Work out the finished part from the listing and answer in its coordinate system (mm). Face numbers are marked on the shaded views. A direction names the side the tool comes from. Round coordinates to 2 decimals unless told otherwise and drop trailing zeros. Loops run counter-clockwise (first coordinate to the right, second up) from the corner with the lowest first, then second, coordinate; pieces in that order, holes last. Notation, with made-up numbers: (35, 23.25) - (64, 23.25) arc R6 ccw to (64, 29.25) - close; hole circle Ø7 at (6.25, -15.5). An arc over 180 degrees is marked (long way). Return JSON: item names as keys, results as strings.
from build123d import *
from build123d.topology import SkipClean

# Parameters (mm, degrees)
EXTRUDE_1_DEPTH     = 3.5
SKETCH_2_R          = 1.25
CUT_EXTRUDE_3_DEPTH = 5.5
SKETCH_3_W          = 20
SKETCH_3_H          = 8
EXTRUDE_2_DEPTH     = 2.886751
SKETCH_4_R          = 1
EXTRUDE_3_DEPTH     = 1


with BuildPart() as part:
    # 草图1 → 凸台-拉伸1 (new, symmetric)
    with BuildSketch(Plane.XY):
        with BuildLine():
            Line((0, 0), (6.245432753, 0))
            ThreePointArc((6.245432753, 0), (6.54659813, -0.100876691), (6.72624124, -0.362802336))
            Line((6.72624124, -0.362802336), (7.280170813, -2.304045596))
            Line((7.280170813, -2.304045596), (3.822659371, -16.095442623))
            Line((3.822659371, -16.095442623), (6.622757346, -16.797428852))
            Line((6.622757346, -16.797428852), (10.080268787, -3.006031824))
            Line((10.080268787, -3.006031824), (8.923233948, 1.048790655))
            ThreePointArc((8.923233948, 1.048790655), (8.204661507, 2.096493237), (7, 2.5))
            Line((7, 2.5), (0, 2.5))
            Line((0, 2.5), (0, 0))
        make_face()
    extrude(amount=EXTRUDE_1_DEPTH, both=True)

    # 草图2 → 切除-拉伸3 (cut)
    with BuildSketch(Plane.XZ):
        with Locations((2.5, 0)):
            Circle(SKETCH_2_R)
    extrude(amount=-CUT_EXTRUDE_3_DEPTH, mode=Mode.SUBTRACT)

    # 草图3 → 凸台-拉伸2 (add)
    with SkipClean():  # the faces are left unmerged after this step: merging them gives an invalid solid
        with BuildSketch(Plane(origin=(10.193230201, -2.555448877, 0), x_dir=(0, 0, -1), z_dir=(0.969982391695105, -0.24317516279719864, 0))):
            with Locations((0, -10.682720116)):
                Rectangle(SKETCH_3_W, SKETCH_3_H)
        extrude(amount=-EXTRUDE_2_DEPTH)

    # 草图4 → 凸台-拉伸3 (add)
    with SkipClean():  # the faces are left unmerged after this step: merging them gives an invalid solid
        with BuildSketch(Plane(origin=(10.193230201, -2.555448877, 0), x_dir=(0, 0, -1), z_dir=(0.969982391695105, -0.24317516279719864, 0))):
            with Locations(Location((-6.050193859, -10.752531826, 0), (0, 0, 270))):
                Circle(SKETCH_4_R)
        extrude_3 = extrude(amount=EXTRUDE_3_DEPTH)

    # 草图5 → 旋转1 (revolve)
    with SkipClean():  # the faces are left unmerged after this step: merging them gives an invalid solid
        with BuildSketch(Plane(origin=(-2.614748677, -10.429766537, 0), x_dir=(-0.969982391695105, 0.24317516279719864, 0), z_dir=(0.24317516279719864, 0.969982391695105, 0))):
            with BuildLine():
                Line((-11.508675506, 6.050193859), (-15.240726313, 6.050193859))
                ThreePointArc((-15.240726313, 6.050193859), (-13.758364403, 7.982045511), (-11.508675506, 7.050193859))
                Line((-11.508675506, 7.050193859), (-11.508675506, 6.050193859))
            make_face()
        revolve_1 = revolve(axis=Axis((8.548463915, -13.228390577, 6.050193859), (0.9699823916951049, -0.24317516279719897, 0)))

    # 镜向1: 凸台-拉伸3, 旋转1 across plane
    with SkipClean():  # the faces are left unmerged after this step: merging them gives an invalid solid
        add(extrude_3.mirror(Plane.XY))
        add(revolve_1.mirror(Plane.XY))


solid = part.part
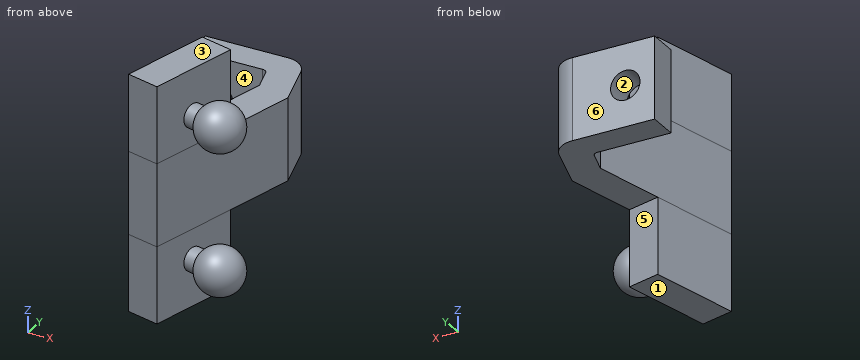
1) Section D-D (x = 5) is taken. Give the vertices of the cut face in (y, z).
Verdict:
{"outline": "(-16.39, -10) - (-11.4, -10) - (-11.4, 3.5) - (-11.4, 10) - (-16.39, 10) - close; (0, -3.5) - (2.5, -3.5) - (2.5, 3.5) - (0, 3.5) - close"}
2) Section A-A (x = 2.5) is taken. Give the vertices of the cut face in (y, z).
Verdict:
{"outline": "(0, -3.5) - (2.5, -3.5) - (2.5, -1.25) - (0, -1.25) - close; (0, 1.25) - (2.5, 1.25) - (2.5, 3.5) - (0, 3.5) - close"}
3) A tool of negligible diameter and unlimited length cuts with its end or side. For the marked faces 5 and 6, from which of +Z, -Z, +X, -X, +Y, -Y can it reach the whole face along a straight path? Write none if from no direction.
Verdict:
{"face 5": "-Z, +X, +Y", "face 6": "+Z, -Z, +X, -X, +Y"}
4) Find the intervals of material crossed by L1, parallel to Z at x = 2.5, y = 1.7; L2, parallel to Z at x = 5.25, y = 0.75; L3, parallel to X at y = -15, z = -7, in increasing order.
Verdict:
{"L1": "z = -3.5 to -1.25, 1.25 to 3.5", "L2": "z = -3.5 to 3.5", "L3": "x = 4.1 to 7.07, 9.1 to 11.36"}
5) Determine the mould class of the marked faces 1, 2, 3 and 4 for opening direction Z: pulls with the +Z half, pulls with the -Z half, needs draft (parallel to the pull), parting line crosses it, or undercut.
Verdict:
{"face 1": "pulls with the -Z half", "face 2": "undercut", "face 3": "pulls with the +Z half", "face 4": "needs draft"}
6) Section C-C (y = -14.75) is taken. Give the vertices of the cut face in (x, z).
Verdict:
{"outline": "(4.16, -10) - (7.14, -10) - (7.14, 10) - (4.16, 10) - close; circle Ø3.34 at (10.23, -6.05); circle Ø3.34 at (10.23, 6.05)"}
7) Flat-ended cylindrical pins translate along their axes: pin 1 (2 mm diameter, centred on x = 6.5, y = -1, fed in from +Z); pin 2 (4 mm diameter, centred on y = -7, z = -4.5, fed in from +X); pin 3 (1.9 mm diameter, centred on x = 2, z = 1.5, fed in from -Y). Find the tip coordinate at first contact, or state that the pin passes through.
Verdict:
{"pin 1": "stops at z = 3.5", "pin 2": "stops at x = 9.51", "pin 3": "stops at y = 0"}
8) Section B-B (z = 0) is taken. Give the vertices of the cut face in (x, y).
Verdict:
{"outline": "(0, 0) - (1.25, 0) - (1.25, 2.5) - (0, 2.5) - close; (3.75, 0) - (6.25, 0) arc R0.5 cw to (6.73, -0.36) - (7.28, -2.3) - (3.82, -16.1) - (6.62, -16.8) - (10.08, -3.01) - (8.92, 1.05) arc R2 ccw to (7, 2.5) - (3.75, 2.5) - close"}
